```python
from build123d import *

# Parameters (mm, degrees)
BOSS_EXTRUDE1_DEPTH = 40
SKETCH2_W           = 30
SKETCH2_H           = 40
BOSS_EXTRUDE2_DEPTH = 130
CUT_EXTRUDE1_DEPTH  = 410


with BuildPart() as part:
    # Sketch1 → Boss-Extrude1 (new body)
    with BuildSketch(Plane.XY):
        Polygon((0, 149.79), (0, 0), (30, 0), (30, 129.79), (319.51, 129.79), (319.51, 0), (349.51, 0), (349.51, 149.79), align=None)
    extrude(amount=BOSS_EXTRUDE1_DEPTH)

    # Sketch2 → Boss-Extrude2 (add)
    with BuildSketch(Plane.XZ.offset(-129.79)):
        with Locations((95, 20)):
            Rectangle(SKETCH2_W, SKETCH2_H)
        with Locations((247.128263463, 20)):
            Rectangle(SKETCH2_W, SKETCH2_H)
    extrude(amount=BOSS_EXTRUDE2_DEPTH)

    # Sketch4 → Cut-Extrude1 (cut)
    with BuildSketch(Plane.ZY):
        with BuildLine():
            ThreePointArc((20, 52.29), (5, 37.29), (20, 22.29))
            Line((20, 22.29), (20, 52.29))
        make_face()
        with BuildLine():
            Line((20, 52.29), (20, 22.29))
            ThreePointArc((20, 22.29), (30.606601718, 26.683398282), (35, 37.29))
            ThreePointArc((35, 37.29), (30.606601718, 47.896601718), (20, 52.29))
        make_face()
    extrude(amount=-CUT_EXTRUDE1_DEPTH, mode=Mode.SUBTRACT)


solid = part.part
```
Could you check a few things on this model? Use its own coordinates, in mm. A direction names the side the tool comes from. Round coordinates to 2 decimals unless told otherwise and drop trailing zeros. Write each loop counter-clockwise with the first axis right and the second up, starting at its lowest first coordinate (ties: lowest second). Pieces come first, ordered by that corner, then holes. Notation, with made-up numbers: M -12,79 L -5,79 A13 cw -5,94 Z; hole C -2,53.25 d10. An arc over 180 degrees is marked long. Answer in a Markdown table with one row per item. Add a question column.
Q1. Imagine slicing it at D-D (x = 72.5). Please give me the cut outline in (y, z), then the cut area to 3 significant figures.
Q2. If I drill on line 1 (X direction, y = 95.5, z = 6); line 2 (Y direction, x = 122, z = 33.5); line 3 (Z direction, x = 104, y = 39), over which ranges is the centre line in solid material (lowest first)? Write a range as from..to.
Q3. On a 3-axis mill with a long thin cutter (end or side, diameter ignored), from which of +Z, -Z, +X, -X, +Y, -Y can I reach the whole of each face in a straight line? I mean faces 1 (the flat face through (80, 66, 20)), 2 (the flat face through (247, -0.21, 20)). Say none if no direction works.
Q4. If we mould it in two halves opening along X, with no side actions, what happens to faces 3 (the flat face through (30, 64, 20)), 4 (the flat face through (290, 129.79, 20)), 5 (the flat face through (95, -0.21, 20)), 6 (the flat face through (0, 76, 20))? For each: +X half, -X half, draft (parallel to the pull), parting line (faces both ways), or undercut.
Q5. Imagine slicing it at B-B (x = 254.5). Please give me the cut outline in (y, z).
Q6. Imagine slicing it at A-A (y = 85). Please give me the cut outline in (x, z).
Q7. Imagine slicing it at C-C (z = 12). Give the number of separate pieces and of enclosed holes in the cut face, then the cut area to 3 significant figures.
Q8. Will these pins go through, and if not, where does the flat tip stop? pin 1 Ø15 at (x, z) = (17, 24.5) entering from -Y; pin 2 Ø12 at (x, z) = (119, 15.5) entering from -Y.
Values:
| question | item | result |
|---|---|---|
| 1 | outline | M 129.79,0 L 149.79,0 L 149.79,40 L 129.79,40 Z |
| 1 | area | 800 mm^2 |
| 2 | line 1 | 0..30, 80..110, 232.13..262.13, 319.51..349.51 |
| 2 | line 2 | 129.79..149.79 |
| 2 | line 3 | 0..5.1, 34.9..40 |
| 3 | face 1 | +Z, -Z, -Y |
| 3 | face 2 | +Z, -Z, +X, -X, -Y |
| 4 | face 3 | undercut |
| 4 | face 4 | undercut |
| 4 | face 5 | draft |
| 4 | face 6 | -X half |
| 5 | outline | M -0.21,0 L 149.79,0 L 149.79,40 L -0.21,40 Z; hole C 37.29,20 d30 |
| 6 | outline | M 0,0 L 30,0 L 30,40 L 0,40 Z; M 80,0 L 110,0 L 110,40 L 80,40 Z; M 232.13,0 L 262.13,0 L 262.13,40 L 232.13,40 Z; M 319.51,0 L 349.51,0 L 349.51,40 L 319.51,40 Z |
| 7 | separate pieces | 5 |
| 7 | enclosed holes | 0 |
| 7 | area | 19,500 mm^2 |
| 8 | pin 1 | y = 0 |
| 8 | pin 2 | y = 129.79 |
